The model under review builds one solid part; all positions refer to its coordinate system, in mm. A direction names the side the tool comes from. Give positions to 0.01 mm unless a question says otherwise; leave off trailing zeros. Order: outer loops, then holes, each group sorted by start corner. A loop starts at its lowest first (then second) coordinate and runs counter-clockwise, first axis right, second up. Notation, with made-up numbers: (70, 41.5) -> (115, 41.5) arc R10 ccw to (115, 55.5) -> close; hole circle Ø10 at (4.25, 89.25). An arc over 180 degrees is marked (long way). Answer as a JSON object with one key per item and string values. Group by question number.
from build123d import *

# Parameters (mm, degrees)
SKETCH1_R           = 3.95
BOSS_EXTRUDE1_DEPTH = 25
CUT_EXTRUDE1_DEPTH  = 25


with BuildPart() as part:
    # Sketch1 → Boss-Extrude1 (new body)
    with BuildSketch(Plane(origin=(0, 0, 0), x_dir=(1, 0, 0), z_dir=(0, 1, 0))):
        with Locations(Location((0, 0, 0), (0, 0, 270))):
            Circle(SKETCH1_R)
    extrude(amount=BOSS_EXTRUDE1_DEPTH)

    # Sketch2 → Cut-Extrude1 (cut)
    with BuildSketch(Plane(origin=(0, 25, 0), x_dir=(1, 0, 0), z_dir=(0, 1, 0))):
        with BuildLine():
            ThreePointArc((-0.25, 2.989565186), (0, 3), (0.25, 2.989565186))
            Line((0.25, 2.989565186), (0.25, 3.942080669))
            Line((0.25, 3.942080669), (-0.25, 3.942080669))
            Line((-0.25, 3.942080669), (-0.25, 2.989565186))
        make_face()
        with BuildLine():
            Line((-3.288942003, -2.187546685), (-2.464039397, -1.711288944))
            ThreePointArc((-2.464039397, -1.711288944), (-2.598076211, -1.5), (-2.714039397, -1.278276242))
            Line((-2.714039397, -1.278276242), (-3.538942003, -1.754533983))
            Line((-3.538942003, -1.754533983), (-3.288942003, -2.187546685))
        make_face()
        with BuildLine():
            Line((3.538942003, -1.754533983), (2.714039397, -1.278276242))
            ThreePointArc((2.714039397, -1.278276242), (2.598076211, -1.5), (2.464039397, -1.711288944))
            Line((2.464039397, -1.711288944), (3.288942003, -2.187546685))
            Line((3.288942003, -2.187546685), (3.538942003, -1.754533983))
        make_face()
    extrude(amount=-CUT_EXTRUDE1_DEPTH, mode=Mode.SUBTRACT)


with BuildPart() as cut_extrude1_kept_piece:
    # of the separate pieces the step leaves, the one the design keeps (cut_extrude1_pieces_kept)
    add(part.part.solids().sort_by_distance((2.464039397, 25, 1.711288944))[0])


solid = cut_extrude1_kept_piece.part
1. For probe 1 along X at (y, z) = (10, -3.5); probe 2 along Z at (x, y) = (-2.75, 14); probe 3 along X at (y, z) = (1.75, 3.25) (3 decimals), list the stretches that pass through material, from the lowest coordinate up. Write a range as [from, to].
2. For pin 1 (1.5 mm diameter, centred on x = 2.5, y = 13.5, fed in from +Z); pin 2 (1 mm diameter, centred on x = 3, y = 6.5, fed in from +Z); pin 3 (3 mm diameter, centred on x = -1, z = -1, fed in from -Y); pin 4 (0.5 mm diameter, centred on y = 13, z = -3.5, fed in from +X) (3 decimals), all flat-tipped, find the tip position at first contact; note any pin that passes through.
3. Take a section at A-A on y = 4.5. Give the boundary of the cut face in (x, z), plus the area to 3 significant figures.
4. Take a section at B-B on z = -0.75. Give the boundary of the cut face in (x, y), plus the area to 3 significant figures.
5. Take a section at C-C on x = 1.5. Give the boundary of the cut face in (y, z), plus the area to 3 significant figures.
6. Draft analysis for pull direction Z (two halves, no side actions). For faces 1 (the cylindrical face through (3.448, 12.325, -1.928)), 2 (the flat face through (3.1, 12.7, 1.5)), 3 (the flat face through (-0.25, 12.7, -3.5)), 4 (the cylindrical face through (-0.05, 12.32, 3.95)), state which applies: pulls with the +Z half, pulls with the -Z half, needs draft (parallel to the pull), parting line crosses it, or undercut.
7. Machinability: for faces 5 (the flat face through (-3.1, 12.7, 1.5)), 6 (the flat face through (0.25, 12.7, -3.5)), 7 (the flat face through (0, 0, 0)), which of the approach directions +Z, -Z, +X, -X, +Y, -Y give a long, thin tool a straight path to every point of the face, cutting with its end or side? Answer none if there is none.
Checks:
{
 "1": {"probe 1": "x = [-1.83, -0.25], [0.25, 1.83]", "probe 2": "z = [-2.84, 1.3], [1.88, 2.84]", "probe 3": "x = [-2.245, 2.245]"},
 "2": {"pin 1": "stops at z = 3.54", "pin 2": "stops at z = 3.06", "pin 3": "stops at y = 0", "pin 4": "stops at x = 2.245"},
 "3": {"outline": "(-3.54, 1.75) arc R3.95 ccw to (-0.25, -3.94) -> (-0.25, -2.99) arc R3 ccw to (0.25, -2.99) -> (0.25, -3.94) arc R3.95 ccw to (3.54, 1.75) -> (2.71, 1.28) arc R3 ccw to (2.46, 1.71) -> (3.29, 2.19) arc R3.95 ccw to (-3.29, 2.19) -> (-2.46, 1.71) arc R3 ccw to (-2.71, 1.28) -> close", "area": "47.6 mm2"},
 "4": {"outline": "(-3.88, 0) -> (3.88, 0) -> (3.88, 25) -> (-3.88, 25) -> close", "area": "194 mm2"},
 "5": {"outline": "(0, -3.65) -> (25, -3.65) -> (25, 3.65) -> (0, 3.65) -> close", "area": "183 mm2"},
 "6": {"face 1": "parting line crosses it", "face 2": "undercut", "face 3": "needs draft", "face 4": "pulls with the +Z half"},
 "7": {"face 5": "+Y, -Y", "face 6": "-Z, +Y, -Y", "face 7": "+Z, -Z, +X, -X, -Y"}
}
